Design review of the part built by this model. Coordinates are the model's own, in mm. A direction names the side the tool comes from. Coordinates: 2 decimals unless noted, no trailing zeros. Order: outer loops, then holes, each group sorted by start corner. A loop starts at its lowest first (then second) coordinate and runs counter-clockwise, first axis right, second up. Notation, with made-up numbers: M -10.5,-13.75 L 1.5,-13.75 A18 ccw 1.5,6.25 Z; hole C 47,29.25 d1. An arc over 180 degrees is marked long. Answer as a JSON object with one key per item and string values.
from build123d import *

# Parameters (mm, degrees)
SKETCH1_W               = 200
SKETCH1_H               = 200
BOSS_EXTRUDE1_DEPTH     = 1000
CUT_EXTRUDE1_DEPTH      = 100
CUT_EXTRUDE1_DEPTH_BACK = 300
SKETCH2_R               = 70
SKETCH3_W               = 100
SKETCH3_H               = 100
CUT_EXTRUDE2_DEPTH      = 100
CUT_EXTRUDE3_DEPTH      = 183
CUT_EXTRUDE3_DEPTH_BACK = 100
SKETCH4_R               = 25
SKETCH5_R               = 50
CUT_EXTRUDE4_DEPTH      = 40
CUT_EXTRUDE5_START      = -40
SKETCH6_R               = 50
CUT_EXTRUDE5_DEPTH      = 40


with BuildPart() as part:
    # Sketch1 → Boss-Extrude1 (new body)
    with BuildSketch(Plane.XY):
        Rectangle(SKETCH1_W, SKETCH1_H)
    extrude(amount=BOSS_EXTRUDE1_DEPTH)

    # Sketch2 → Cut-Extrude1 (cut, two sides: drawn at the far end of the back side and taken through both)
    with BuildSketch(Plane(origin=(100, 0, 0), x_dir=(0, 0, -1), z_dir=(1, 0, 0)).offset(-CUT_EXTRUDE1_DEPTH_BACK)):
        with Locations(Location((-100, 0, 0), (0, 0, 180))):
            Circle(SKETCH2_R)
    extrude(amount=CUT_EXTRUDE1_DEPTH + CUT_EXTRUDE1_DEPTH_BACK, mode=Mode.SUBTRACT)

    # Sketch3 → Cut-Extrude2 (cut)
    with BuildSketch(Plane.XY.offset(1000)):
        Rectangle(SKETCH3_W, SKETCH3_H)
    extrude(amount=-CUT_EXTRUDE2_DEPTH, mode=Mode.SUBTRACT)

    # Sketch4 → Cut-Extrude3 (cut, two sides: drawn at the far end of the back side and taken through both)
    with BuildSketch(Plane(origin=(0, -50, 0), x_dir=(1, 0, 0), z_dir=(0, 1, 0)).offset(-CUT_EXTRUDE3_DEPTH_BACK)):
        with Locations((0, -950)):
            Circle(SKETCH4_R)
    extrude(amount=CUT_EXTRUDE3_DEPTH + CUT_EXTRUDE3_DEPTH_BACK, mode=Mode.SUBTRACT)

    # Sketch5 → Cut-Extrude4 (cut)
    with BuildSketch(Plane(origin=(100, 0, 0), x_dir=(0, 0, -1), z_dir=(1, 0, 0))):
        with Locations((-750, 0)):
            Circle(SKETCH5_R)
    extrude(amount=-CUT_EXTRUDE4_DEPTH, mode=Mode.SUBTRACT)

    # Sketch6 → Cut-Extrude5 (cut)
    with BuildSketch(Plane.ZY.offset(100).offset(CUT_EXTRUDE5_START)):
        with Locations(Location((750, 0, 0), (0, 0, 180))):
            Circle(SKETCH6_R)
    extrude(amount=CUT_EXTRUDE5_DEPTH, mode=Mode.SUBTRACT)


solid = part.part
1) Tool access review of faces 4 (the flat face through (-50, -1, 951)), 5 (the cylindrical face through (-1.4, 42.594, 44.45)), 6 (the cylindrical face through (11.5, 74.6, 972.2)), 7 (the cylindrical face through (-79.72, -15.02, 702.31)), 8 (the flat face through (60, 1, 751)): name each direction out of +Z, -Z, +X, -X, +Y, -Y from which nothing blocks a thin tool from reaching the whole face with its end or side.
Taken from the geometry:
{"face 4": "+Z", "face 5": "+X, -X", "face 6": "+Y, -Y", "face 7": "-X", "face 8": "+X"}
2) Add section D-D (x = 41). State the section outline as (y, z) points, and give its area (3 significant figures).
Taken from the geometry:
{"outline": "M -100,0 L 100,0 L 100,1000 L 50,1000 L 50,900 L -50,900 L -50,1000 L -100,1000 Z; hole C 0,100 d140", "area": "175,000 mm2"}
3) Insertion check: pin 1 Ø10 at (x, y) = (0.5, -69.5) entering from -Z. The pin has a flat end and moves straight along its axis. Give the tip position at first contact, or say it passes through.
Taken from the geometry:
{"pin 1": "stops at z = 0"}
4) To check wall thickness, follow L1, parallel to Z at x = 0, y = 73; L2, parallel to Y at x = 72.5, z = 750. State the ranges of each line that lie inside material, in increasing order.
Taken from the geometry:
{"L1": "z = 0 to 925, 975 to 1000", "L2": "y = -100 to -50, 50 to 100"}
5) Add section C-C (y = 0). State the section outline as (x, z) points.
Taken from the geometry:
{"outline": "M -100,0 L 100,0 L 100,30 L -100,30 Z; M -100,170 L 100,170 L 100,700 L 60,700 L 60,800 L 100,800 L 100,1000 L 50,1000 L 50,900 L -50,900 L -50,1000 L -100,1000 L -100,800 L -60,800 L -60,700 L -100,700 Z"}
6) Add section B-B (z = 950). State the section outline as (x, y) points.
Taken from the geometry:
{"outline": "M -100,-100 L -25,-100 L -25,-50 L -50,-50 L -50,50 L -25,50 L -25,100 L -100,100 Z; M 25,-100 L 100,-100 L 100,100 L 25,100 L 25,50 L 50,50 L 50,-50 L 25,-50 Z"}
7) Mouldability with a two-part tool opening along X and no side actions: class faces 1 (the flat face through (-60, -1, 751)), 2 (the flat face through (-1, 100, 493)), 3 (the flat face through (-1, 1, 900)) as released by +X, released by -X, zero draft, split by the parting line, or undercut.
Taken from the geometry:
{"face 1": "released by -X", "face 2": "zero draft", "face 3": "undercut"}
8) Add section A-A (x = -1). State the section outline as (y, z) points, and give its area (3 significant figures).
Taken from the geometry:
{"outline": "M -100,0 L 100,0 L 100,925.02 L 50,925.02 L 50,900 L -50,900 L -50,925.02 L -100,925.02 Z; M -100,974.98 L -50,974.98 L -50,1000 L -100,1000 Z; M 50,974.98 L 100,974.98 L 100,1000 L 50,1000 Z; hole C 0,100 d140", "area": "170,000 mm2"}
